Work out the finished part from the listing and answer in its coordinate system (mm). A direction names the side the tool comes from. Round coordinates to 2 decimals unless told otherwise and drop trailing zeros. Loops run counter-clockwise (first coordinate to the right, second up) from the corner with the lowest first, then second, coordinate; pieces in that order, holes last. Notation, with made-up numbers: (70, 47) - (117, 47) arc R15 cw to (117, 51) - close; hole circle Ø10 at (-34, -20.5). An arc over 180 degrees is marked (long way). Answer as CSV lines item,"result". Start each with the question number.
```python
from build123d import *

# Parameters (mm, degrees)
ESTRUSIONE_ESTRUSIONE1_DEPTH = 120
TAGLIO_ESTRUSIONE2_REACH     = 82
SCHIZZO6_R                   = 7.75
TAGLIO_ESTRUSIONE3_REACH     = 82
SCHIZZO7_R                   = 11.5
M4_TAPPED_HOLE1_D            = 3.3
SCHIZZO12_R                  = 3
TAGLIO_ESTRUSIONE4_DEPTH     = 10
SCHIZZO14_R                  = 2.6
TAGLIO_ESTRUSIONE5_DEPTH     = 10
SMUSSO2_SIZE                 = 1
FORO_FILETTATO_M3_1_D        = 2.5
FORO_FILETTATO_M3_1_DEPTH    = 10
FORO_FILETTATO_M3_1_TIP      = 0.751075774


with BuildPart() as part:
    # Schizzo1 → Estrusione-Estrusione1 (new body)
    with BuildSketch(Plane.XY):
        Polygon((0, 0), (-80, 0), (-80, -8), (-8, -8), (-8, -80), (0, -80), align=None)
    extrude(amount=ESTRUSIONE_ESTRUSIONE1_DEPTH)

    # Schizzo6 → Taglio-Estrusione2 (cut, up to next)
    with BuildSketch(Plane(origin=(0, 0, 0), x_dir=(1, 0, 0), z_dir=(0, 1, 0)), mode=Mode.PRIVATE) as taglio_estrusione2_sk1:
        with Locations((-23, -21.5)):
            Circle(SCHIZZO6_R)
    taglio_estrusione2_tool1 = extrude(taglio_estrusione2_sk1.sketch, amount=-TAGLIO_ESTRUSIONE2_REACH, mode=Mode.PRIVATE) & part.part
    add(taglio_estrusione2_tool1.solids().sort_by_distance((-23, 0, 21.5))[0], mode=Mode.SUBTRACT)
    # Schizzo6 → Taglio-Estrusione2 (cut, up to next)
    with BuildSketch(Plane(origin=(0, 0, 0), x_dir=(1, 0, 0), z_dir=(0, 1, 0)), mode=Mode.PRIVATE) as taglio_estrusione2_sk2:
        with Locations((-23, -98.5)):
            Circle(SCHIZZO6_R)
    taglio_estrusione2_tool2 = extrude(taglio_estrusione2_sk2.sketch, amount=-TAGLIO_ESTRUSIONE2_REACH, mode=Mode.PRIVATE) & part.part
    add(taglio_estrusione2_tool2.solids().sort_by_distance((-23, 0, 98.5))[0], mode=Mode.SUBTRACT)

    # Schizzo7 → Taglio-Estrusione3 (cut, up to next)
    with BuildSketch(Plane(origin=(0, 0, 0), x_dir=(1, 0, 0), z_dir=(0, 1, 0)), mode=Mode.PRIVATE) as taglio_estrusione3_sk1:
        with Locations((-29, -60)):
            Circle(SCHIZZO7_R)
    taglio_estrusione3_tool1 = extrude(taglio_estrusione3_sk1.sketch, amount=-TAGLIO_ESTRUSIONE3_REACH, mode=Mode.PRIVATE) & part.part
    add(taglio_estrusione3_tool1.solids().sort_by_distance((-29, 0, 60))[0], mode=Mode.SUBTRACT)

    # M4 Tapped Hole1 (through all)
    with Locations(Plane(origin=(0, 0, 0), x_dir=(1, 0, 0), z_dir=(0, 1, 0))):
        with Locations((-29, -44.5), (-44.5, -60), (-29, -75.5), (-13.5, -60), (-29, -60)):
            Hole(M4_TAPPED_HOLE1_D / 2)

    # Schizzo12 → Taglio-Estrusione4 (cut)
    with BuildSketch(Plane(origin=(0, 0, 0), x_dir=(0, 0, -1), z_dir=(1, 0, 0))):
        with Locations((-113.75, -19)):
            Circle(SCHIZZO12_R)
        with Locations((-83.25, -19)):
            Circle(SCHIZZO12_R)
        with Locations((-36.75, -19)):
            Circle(SCHIZZO12_R)
        with Locations((-6.25, -19)):
            Circle(SCHIZZO12_R)
        with Locations((-83.25, -69)):
            Circle(SCHIZZO12_R)
        with Locations((-113.75, -69)):
            Circle(SCHIZZO12_R)
        with Locations((-6.25, -69)):
            Circle(SCHIZZO12_R)
        with Locations((-36.75, -69)):
            Circle(SCHIZZO12_R)
    extrude(amount=-TAGLIO_ESTRUSIONE4_DEPTH, mode=Mode.SUBTRACT)

    # Schizzo14 → Taglio-Estrusione5 (cut)
    with BuildSketch(Plane(origin=(0, 0, 0), x_dir=(1, 0, 0), z_dir=(0, 1, 0))):
        with Locations((-70, -18)):
            Circle(SCHIZZO14_R)
        with Locations((-70, -60)):
            Circle(SCHIZZO14_R)
        with Locations((-70, -102)):
            Circle(SCHIZZO14_R)
        with Locations((-55, -35)):
            Circle(SCHIZZO14_R)
        with Locations((-55, -85)):
            Circle(SCHIZZO14_R)
    extrude(amount=-TAGLIO_ESTRUSIONE5_DEPTH, mode=Mode.SUBTRACT)

    # Smusso2
    smusso2_edges = [part.edges().sort_by_distance(p)[0] for p in [
        (-40.5, 0, 60),
    ]]
    chamfer(smusso2_edges, length=SMUSSO2_SIZE)

    # Foro filettato M3-1
    with Locations(Plane.XY.offset(120)):
        with Locations((-10, -4), (-29, -4)):
            Hole(FORO_FILETTATO_M3_1_D / 2, depth=FORO_FILETTATO_M3_1_DEPTH)
            with Locations((0, 0, -(FORO_FILETTATO_M3_1_DEPTH + FORO_FILETTATO_M3_1_TIP / 2))):  # 118° drill point
                Cone(0, FORO_FILETTATO_M3_1_D / 2, FORO_FILETTATO_M3_1_TIP, mode=Mode.SUBTRACT)


solid = part.part
```
Item 1: Determine the mould class of faces 1 (the face through (-3.944, -18.868, 39.747)), 2 (the face through (-27.784, -4.056, 43.385)), 3 (the face through (-8, -43, 59)) for opening direction X: pulls with the +X half, pulls with the -X half, needs draft (parallel to the pull), parting line crosses it, or undercut.
Item 2: Find the intervals of material crossed by L1, parallel to Z at x = -55, y = -4; L2, parallel to X at y = -5.25, z = 60; L3, parallel to Y at x = -2, z = 113, in increasing order.
Item 3: Section A-A, the plane y = -19 is taken. Give the vertices of the cut face in (x, z).
Item 4: Which of the six approach directions +Z, -Z, +X, -X, +Y, -Y give full straight-line access (tool end or side, diameter ignored) to faces 4 (the face through (-30.155, -4.479, 114.93)), 5 (the face through (-56.916, -3.944, 83.243))?
Item 5: Section C-C, the plane y = -61 is taken. Give the vertices of the cut face in (x, z).
Item 6: Section B-B, the plane x = -44.5 is taken. Give the vertices of the cut face in (y, z).
Item 7: Flat-ended cylindrical pins translate along their axes: pin 1 Ø7 at (y, z) = (-69, 6.25) entering from +X; pin 2 Ø1.5 at (x, z) = (-30.5, 74.5) entering from -Y; pin 3 Ø8 at (y, z) = (-30, 40) entering from -X; pin 4 Ø2 at (x, y) = (-10, -4) entering from +Z. Find the tip coordinate at first contact, or state that the pin passes through.
Answer:
1,face 1,"needs draft"
1,face 2,"undercut"
1,face 3,"pulls with the -X half"
2,L1,"z = 0 to 32.4, 37.6 to 82.4, 87.6 to 120"
2,L2,"x = -80 to -72.6, -67.4 to -46.15, -42.85 to -40.5, -17.5 to -15.15, -11.85 to 0"
2,L3,"y = -80 to -71.9, -66.1 to -21.9, -16.1 to 0"
3,outline,"(-8, 0) - (0, 0) - (0, 3.25) - (-8, 3.25) - close; (-8, 9.25) - (0, 9.25) - (0, 33.75) - (-8, 33.75) - close; (-8, 39.75) - (0, 39.75) - (0, 80.25) - (-8, 80.25) - close; (-8, 86.25) - (0, 86.25) - (0, 110.75) - (-8, 110.75) - close; (-8, 116.75) - (0, 116.75) - (0, 120) - (-8, 120) - close"
4,face 4,"+Z"
4,face 5,"+Y, -Y"
5,outline,"(-8, 0) - (0, 0) - (0, 120) - (-8, 120) - close"
6,outline,"(-8, 0) - (0, 0) - (0, 58.35) - (-8, 58.35) - close; (-8, 61.65) - (0, 61.65) - (0, 120) - (-8, 120) - close"
7,pin 1,"stops at x = 0"
7,pin 2,"stops at y = -8"
7,pin 3,"stops at x = -8"
7,pin 4,"stops at z = 109.85"
